Design review of the part built by this model. Coordinates are the model's own, in mm. Face numbers are marked on the shaded views. A direction names the side the tool comes from. Round coordinates to 2 decimals unless told otherwise and drop trailing zeros. Order: outer loops, then holes, each group sorted by start corner. A loop starts at its lowest first (then second) coordinate and runs counter-clockwise, first axis right, second up.
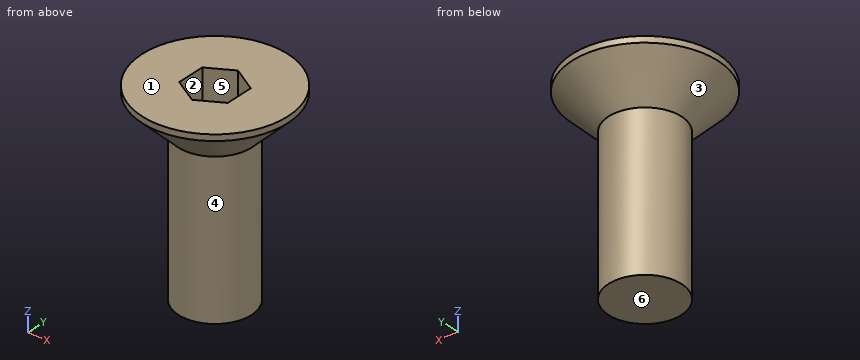
Autodesk Inventor part; units mm, degrees
ref_plane "YZ Plane" through (0, 0, 0) normal (1, 0, 0) x (0, 1, 0)
ref_plane "XZ Plane" through (0, 0, 0) normal (0, 1, 0) x (-1, 0, 0)
ref_plane "XY Plane" through (0, 0, 0) normal (0, 0, 1) x (1, 0, 0)
sketch "スケッチ1" plane through (0, 0, 0) normal (0, 0, 1) x (1, 0, 0)
  circle A0 centre (0, 0) radius 1.5
  dimension "d0" = 3
extrude "押し出し1" add sketch "スケッチ1" along normal blind 8
thread "ねじ1"
sketch "スケッチ2" plane through (0, 0, 8) normal (0, 0, 1) x (1, 0, 0)
  circle A0 centre (0, 0) radius 3
  dimension "d5" = 6
extrude "押し出し2" add sketch "スケッチ2" against normal blind 1.75
chamfer "面取り1" distance 1.5 angle 45 1 edges at (-3, 0, 6.25)
sketch "スケッチ3" plane through (0, 0, 8) normal (0, 0, 1) x (1, 0, 0)
  line L0 (0, 1.1547) -> (1, 0.5774)
  line L1 (1, 0.5774) -> (1, -0.5774)
  line L2 (1, -0.5774) -> (0, -1.1547)
  line L3 (0, -1.1547) -> (-1, -0.5774)
  line L4 (-1, -0.5774) -> (-1, 0.5774)
  line L5 (-1, 0.5774) -> (0, 1.1547)
  point P0 (0, 0)
  point P1 (0, 0)
  dimension "d11" = 2
extrude "押し出し3" cut sketch "スケッチ3" against normal blind 1.5
properties part number "m3皿ネジ8" material "鉄 灰色"
1) Take a section at B-B on z = 7.25. Give the boundary of the cut face in (x, y).
Results:
outline: circle Ø5 at (0, 0); hole (-1, -0.58) - (0, -1.15) - (1, -0.58) - (1, 0.58) - (0, 1.15) - (-1, 0.58) - close
2) Take a section at C-C on z = 5.75. Give the boundary of the cut face in (x, y), plus the area to 3 significant figures.
Results:
outline: circle Ø3 at (0, 0)
area: 7.07 mm2
3) For the marked faces 4, 5 and 6, list the 3-axis set-ups (+Z, -Z, +X, -X, +Y, -Y) from which the entire face can be reached by the end or side of a thin tool; tool diameter is ignored.
Results:
face 4: -Z
face 5: +Z
face 6: -Z, +X, -X, +Y, -Y
4) The part is to be moulded in two halves that separate along Y. For the marked faces 1, 2 and 3, say which applies: released by +Y, released by -Y, zero draft, split by the parting line, or undercut.
Results:
face 1: zero draft
face 2: undercut
face 3: split by the parting line
5) To check wall thickness, follow line 1 along X through (y, z) = (-1.05, 7.5); line 2 along Z through (x, y) = (-0.65, 0.1); line 3 along Y through (x, z) = (0, 2.5). State the ranges of each line that lie inside material, in increasing order.
Results:
line 1: x = -2.54 to -0.18, 0.18 to 2.54
line 2: z = 0 to 6.5
line 3: y = -1.5 to 1.5
6) Clearance check with flat-ended pins moving along their axes: P1, Ø1.5, axis at x = -2, z = 3.5, coming from the -Y side; P2, Ø1.5, axis at x = 0.5, y = 0.5, coming from the -Z side; P3, Ø1, axis at x = 1.5, z = 3, coming from the +Y side; P4, Ø1.5, axis at x = 1.5, z = 4, coming from the -Y side. State where each tip first meets the part, or that it passes through.
Results:
P1: stops at y = -0.83
P2: stops at z = 0
P3: stops at y = 1.12
P4: stops at y = -1.3
